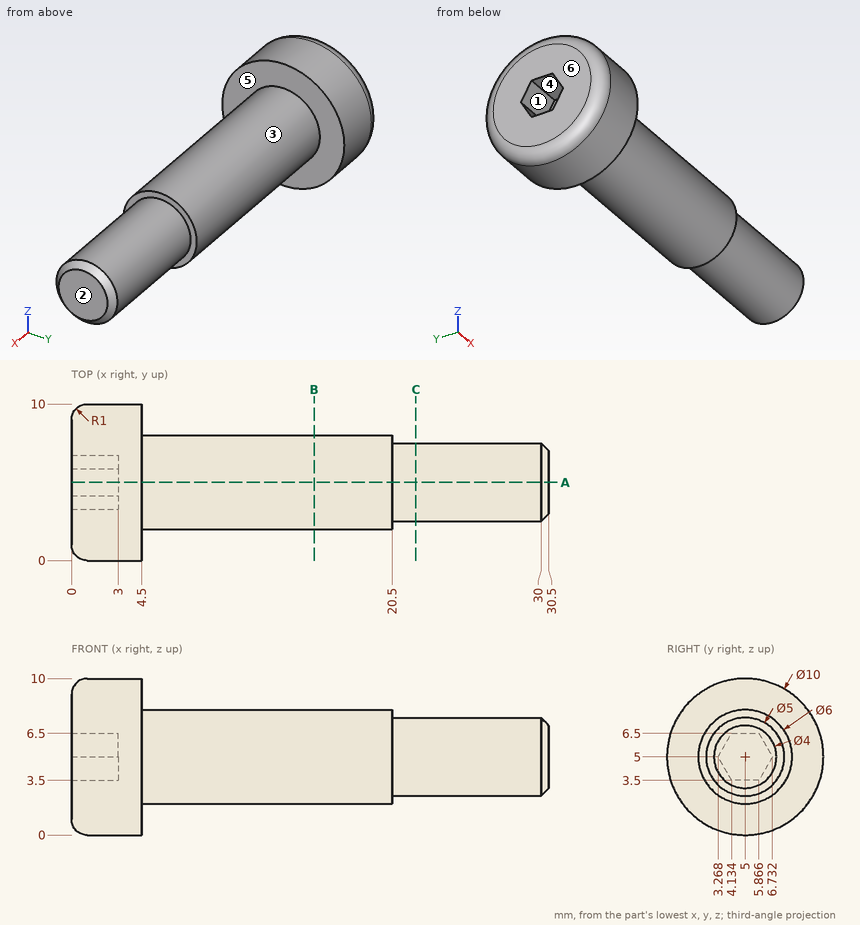
Geometry check sheet. Reference: drawing and pictorial views, mm from the part's lowest x, y, z. A direction names the side the tool comes from. Coordinates: 2 decimals unless noted, no trailing zeros. Write each loop counter-clockwise with the first axis right and the second up, starting at its lowest first coordinate (ties: lowest second). Pieces come first, ordered by that corner, then holes. Notation, with made-up numbers: M 5.25,7.25 L 16.25,7.25 A24 cw 16.25,31.25 Z; hole C 28,52.25 d11. An arc over 180 degrees is marked long. Write item = value, one per line. Start each with the question number.
1. Tool access check on the marked faces 5 and 6. Record the directions out of +Z, -Z, +X, -X, +Y, -Y that give a thin tool (end or side, any length) a straight path to the whole face; none if there is none.
2. Mould release check, pull along Y, two halves, no side actions. Record for the marked faces 1, 2, 3 and 4: pulls with the +Y half, pulls with the -Y half, needs draft (parallel to the pull), parting line crosses it, or undercut.
3. Sectioned sample at B-B (x = 15.5). Record the cut outline in (y, z), then the cut area to 3 significant figures.
4. Sectioned sample at C-C (x = 22). Record the cut outline in (y, z), then the cut area to 3 significant figures.
5. Go/stop test with flat-tipped pins: pin 1 (4 mm diameter, centred on x = 11, y = 2, fed in from -Z); pin 2 (1.5 mm diameter, centred on x = 25.5, y = 4, fed in from -Z); pin 3 (6 mm diameter, centred on x = 14.5, y = 7, fed in from +Z). Record where each tip stops, or that it passes through.
6. Sectioned sample at A-A (y = 5). Record the cut outline in (x, z).
7. Thickness scan on probe 1 along Z at (x, y) = (22, 3.5); probe 2 along X at (y, z) = (1.5, 5.75). Record the ranges inside material, lowest first.
The answers:
q1.face_5 = +X
q1.face_6 = +Z, -Z, -X, +Y, -Y
q2.face_1 = undercut
q2.face_2 = needs draft
q2.face_3 = parting line crosses it
q2.face_4 = undercut
q3.outline = C 5,5 d6
q3.area = 28.3 mm²
q4.outline = C 5,5 d5
q4.area = 19.6 mm²
q5.pin_1 = 2.17
q5.pin_2 = 2.51
q5.pin_3 = 8
q6.outline = M 0,1 A1 ccw 1,0 L 4.5,0 L 4.5,2 L 20.5,2 L 20.5,2.5 L 30,2.5 L 30.5,3 L 30.5,7 L 30,7.5 L 20.5,7.5 L 20.5,8 L 4.5,8 L 4.5,10 L 1,10 A1 ccw 0,9 L 0,6.5 L 3,6.5 L 3,3.5 L 0,3.5 Z
q7.probe_1 = 3 to 7
q7.probe_2 = 0 to 4.5
